Geometry check sheet. Reference: drawing and pictorial views, mm from the part's lowest x, y, z. A direction names the side the tool comes from. Give positions to 0.01 mm unless a question says otherwise; leave off trailing zeros. Order: outer loops, then holes, each group sorted by start corner. A loop starts at its lowest first (then second) coordinate and runs counter-clockwise, first axis right, second up.
Item 1: Access from +Z, -Z, +X, -X, +Y, -Y to the whole of each face (thin tool, end or side, straight path). Record for the marked faces 1 and 2.
Item 2: Sectioned sample at D-D on x = 30.15. Record the boundary of the cut face in (y, z), and give its area (3 significant figures).
Item 3: Sectioned sample at A-A on z = 14. Record the boundary of the cut face in (x, y).
Item 4: Material ranges on line 1 along X through (y, z) = (0.6, 14); line 2 along X through (y, z) = (0.6, 7); line 3 along Z through (x, y) = (30.15, 0.85), recorded low to high.
Item 5: Sectioned sample at C-C on y = 21.5. Record the boundary of the cut face in (x, z), and give its area (3 significant figures).
Item 6: Gauge pin test, flat ends, axial feed: P1, Ø6, axis at x = 47.5, z = 9.5, coming from the +Y side; P2, Ø0.8, axis at y = 20.5, z = 27.5, coming from the +X side; P3, Ø1.1, axis at y = 23.5, z = 27.5, coming from the -X side. Record the tip position at first contact, or that the pin passes through.
Item 7: Sectioned sample at B-B on x = 4.15. Record the boundary of the cut face in (y, z), and give its area (3 significant figures).
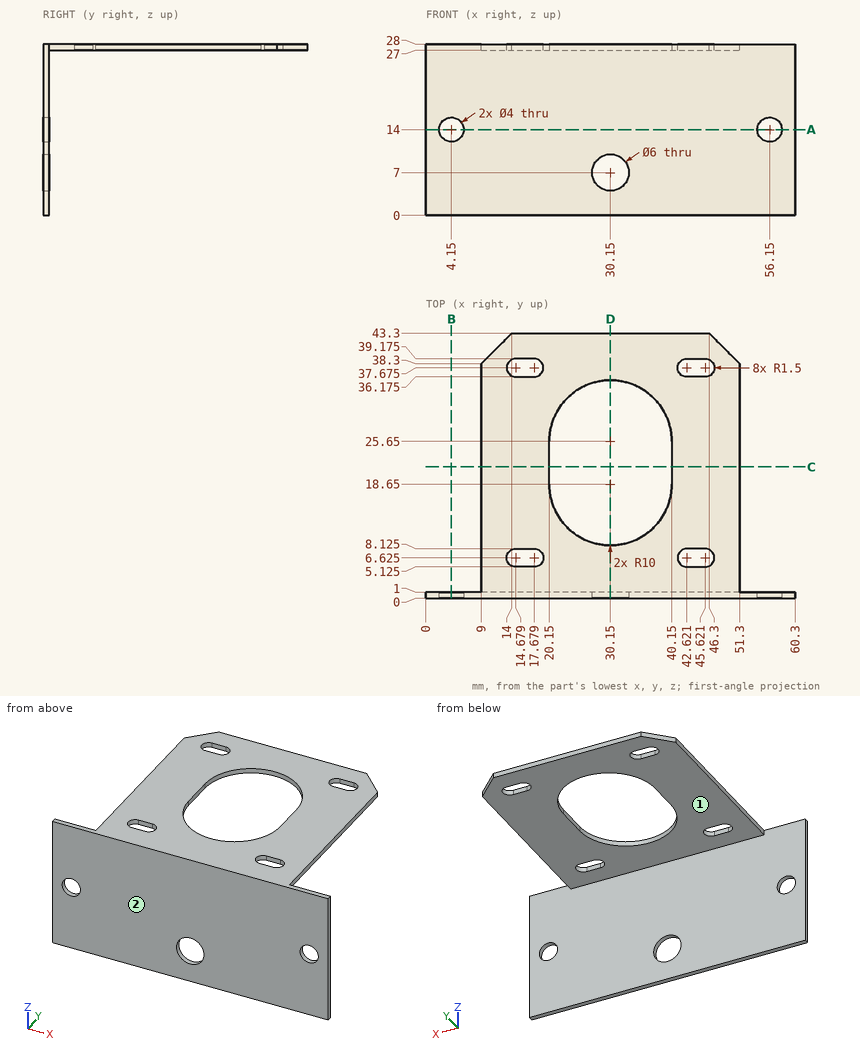
Report:
1. face 1: -Z, +X, -X, +Y
1. face 2: +Z, -Z, +X, -X, -Y
2. outline: (0, 0) - (1, 0) - (1, 4) - (0, 4) - close; (0, 10) - (1, 10) - (1, 27) - (8.65, 27) - (8.65, 28) - (0, 28) - close; (35.65, 27) - (43.3, 27) - (43.3, 28) - (35.65, 28) - close
2. area: 37.3 mm2
3. outline: (0, 0) - (2.15, 0) - (2.15, 1) - (0, 1) - close; (6.15, 0) - (54.15, 0) - (54.15, 1) - (6.15, 1) - close; (58.15, 0) - (60.3, 0) - (60.3, 1) - (58.15, 1) - close
4. line 1: x = 0 to 2.15, 6.15 to 54.15, 58.15 to 60.3
4. line 2: x = 0 to 27.15, 33.15 to 60.3
4. line 3: z = 0 to 4, 10 to 28
5. outline: (9, 27) - (20.15, 27) - (20.15, 28) - (9, 28) - close; (40.15, 27) - (51.3, 27) - (51.3, 28) - (40.15, 28) - close
5. area: 22.3 mm2
6. P1: stops at y = 1
6. P2: stops at x = 51.3
6. P3: stops at x = 9
7. outline: (0, 0) - (1, 0) - (1, 12) - (0, 12) - close; (0, 16) - (1, 16) - (1, 28) - (0, 28) - close
7. area: 24.0 mm2
